```python
from build123d import *

# Parameters (mm, degrees)
BOSS_EXTRUDE1_DEPTH = 2.6
FILLET1_R           = 0.5
BOSS_EXTRUDE2_DEPTH = 0.4


with BuildPart() as part:
    # Sketch4 → Boss-Extrude1 (new body)
    with BuildSketch(Plane.XY):
        with BuildLine():
            add(Edge.make_bspline(
                [(0, 4), (0.515028324, 2.414905806), (1.36313107, 0.834026377), (3, 0)],
                knots=[0, 0, 0, 0, 1, 1, 1, 1], degree=3))
            add(Edge.make_bspline(
                [(0, -4), (0.515028324, -2.414905806), (1.36313107, -0.834026377), (3, 0)],
                knots=[0, 0, 0, 0, 1, 1, 1, 1], degree=3))
            add(Edge.make_bspline(
                [(0, -4), (-0.515028324, -2.414905806), (-1.36313107, -0.834026377), (-3, 0)],
                knots=[0, 0, 0, 0, 1, 1, 1, 1], degree=3))
            add(Edge.make_bspline(
                [(0, 4), (-0.515028324, 2.414905806), (-1.36313107, 0.834026377), (-3, 0)],
                knots=[0, 0, 0, 0, 1, 1, 1, 1], degree=3))
        make_face()
    extrude(amount=BOSS_EXTRUDE1_DEPTH)

    # Fillet1
    fillet1_edges = [part.edges().sort_by_distance(p)[0] for p in [
        (0, -4, 1.3),
        (-3, 0, 1.3),
        (3, 0, 1.3),
        (0, 4, 1.3),
    ]]
    fillet(fillet1_edges, radius=FILLET1_R)

    # Sketch5 → Boss-Extrude2 (add)
    with BuildSketch(Plane.XY):
        with BuildLine():
            ThreePointArc((-2.929739435, 1.212558746), (-3.546732478, 0), (-2.929739435, -1.212558746))
            add(Edge.make_bspline(
                [(-2.929739435, -1.212558746), (-2.754213175, -1.340380107), (-2.591067356, -1.481611947), (-2.286979377, -1.788126606), (-2.14580641, -1.953887397), (-1.757808942, -2.473821282), (-1.543643929, -2.852932461), (-1.361963313, -3.246613691)],
                knots=[0, 0, 0, 0, 0.25, 0.25, 0.5, 0.5, 1, 1, 1, 1], degree=3))
            ThreePointArc((-1.361963313, -3.246613691), (0, -4.118078938), (1.361963313, -3.246613691))
            add(Edge.make_bspline(
                [(1.361963313, -3.246613691), (1.543598049, -2.853031879), (1.757635539, -2.47411695), (2.274781933, -1.780991218), (2.578788315, -1.468127627), (2.929739435, -1.212558746)],
                knots=[0, 0, 0, 0, 0.5, 0.5, 1, 1, 1, 1], degree=3))
            ThreePointArc((2.929739435, -1.212558746), (3.546732478, 0), (2.929739435, 1.212558746))
            add(Edge.make_bspline(
                [(2.929739435, 1.212558746), (2.754213175, 1.340380107), (2.591067356, 1.481611947), (2.286979377, 1.788126606), (2.14580641, 1.953887397), (1.757808942, 2.473821282), (1.543643929, 2.852932461), (1.361963313, 3.246613691)],
                knots=[0, 0, 0, 0, 0.25, 0.25, 0.5, 0.5, 1, 1, 1, 1], degree=3))
            ThreePointArc((1.361963313, 3.246613691), (0, 4.118078938), (-1.361963313, 3.246613691))
            add(Edge.make_bspline(
                [(-1.361963313, 3.246613691), (-1.543598049, 2.853031879), (-1.757635539, 2.47411695), (-2.274781933, 1.780991218), (-2.578788315, 1.468127627), (-2.929739435, 1.212558746)],
                knots=[0, 0, 0, 0, 0.5, 0.5, 1, 1, 1, 1], degree=3))
        make_face()
    extrude(amount=BOSS_EXTRUDE2_DEPTH)


solid = part.part
```
Source: CAD feature listing. Evaluate the final solid. Frame: model axes, mm. A direction names the side the tool comes from. Give positions to 0.01 mm unless a question says otherwise; leave off trailing zeros. Use a Markdown table: item, result. Add a question column.
(1) Ray query, line 1 (Z direction, x = 0.75, y = -2.5); line 2 (X direction, y = 0, z = 1.45); line 3 (X direction, y = -2.5, z = 2). Return the intervals inside material, ascending.
(2) First-contact query: pin 1 Ø1 at (x, z) = (2, 1) entering from -Y; pin 2 Ø1.5 at (y, z) = (2, 1.5) entering from -X; pin 3 Ø1 at (y, z) = (0, 1) entering from +X. Flat tips, straight axial feed; report the tip coordinate or a pass-through.
(3) Access query for faces 1 (the face through (2, 1, 0.4)), 2 (the face through (0.024, 4.118, 0.197)). Directions: +Z, -Z, +X, -X, +Y, -Y. A direction counts if a zero-diameter tool reaches every point of the face in a straight line with its end or side. Return the directions, or none.
Checked values:
| question | item | result |
|---|---|---|
| 1 | line 1 | 0 to 0.4 |
| 1 | line 2 | -2.55 to 2.55 |
| 1 | line 3 | -0.61 to 0.61 |
| 2 | pin 1 | y = -1.18 |
| 2 | pin 2 | x = -1.44 |
| 2 | pin 3 | x = 2.55 |
| 3 | face 1 | +Z |
| 3 | face 2 | +Z, -Z, +Y |
